Part model, mm, in its own coordinate system. A direction names the side the tool comes from. Round coordinates to 2 decimals unless told otherwise and drop trailing zeros. Write each loop counter-clockwise with the first axis right and the second up, starting at its lowest first coordinate (ties: lowest second). Pieces come first, ordered by that corner, then holes. Notation, with made-up numbers: M -20.5,53.5 L 9.5,53.5 A17 ccw 9.5,62.5 Z; hole C -18,56.25 d11. An arc over 180 degrees is marked long. One line per question, with ' | ' between items. Start each with the question number.
1) Saw through at A-A (y = 97). List the corners of the cut face in (x, z).
2) Saw through at B-B (z = 91.5). List the corners of the cut face in (x, y), plus the area to 3 significant figures.
3) Mould opens along Y. For faces 5 (the face through (110.68, -160.09, 123.18)), 6 (the face through (-1, 158, 124.46)), 7 (the face through (-2, -165.1, 2)) say: pulls with the +Y half, pulls with the -Y half, needs draft (parallel to the pull), parting line crosses it, or undercut.
4) Saw through at C-C (x = 38.5). List the corners of the cut face in (y, z).
5) Drop flat-ended pins along their axis: pin 1 Ø3 at (y, z) = (-39, 125.5) entering from +X; pin 2 Ø1.4 at (x, y) = (112.5, -5) entering from +Z; pin 3 Ø8 at (x, y) = (75, 66) entering from +Z. Give the stop position or say it passes through.
6) Tool access for faces 1 (the face through (-98, -151.1, 125.6)), 2 (the face through (-103.06, -151.12, -45.68)), 3 (the face through (1, 159, 127)), 4 (the face through (110.68, 159.95, 123.18)): list every direction of +Z, -Z, +X, -X, +Y, -Y with a clear straight run to the whole face (end or side of a thin tool).
7) Wall check: probe 1 along Y at (x, z) = (77.5, -93); probe 2 along X at (y, z) = (-65, -15.5); probe 3 along X at (y, z) = (69.5, 112.5). Give the ranges that are in metal, low to high. Write a range as [from, to].
```python
from build123d import *

# Parameters (mm, degrees)
F1_DEPTH      = 165.1
F1_DEPTH_BACK = 165.1
F3_DEPTH      = 12.7
F5_DEPTH      = 5.08
F7_DEPTH      = 5.08
F8_W          = 223.52
F8_H          = 5.08
F9_DEPTH      = 320.04
F11_DEPTH     = 25.4


with BuildPart() as f1:
    # F0 (on Front) → F1 (new body, two sides)
    with BuildSketch(Plane.XZ) as f1_sk:
        with BuildLine():
            Line((-101.6, -127), (101.6, -127))
            ThreePointArc((101.6, -127), (110.580256, -123.280256), (114.3, -114.3))
            Line((114.3, -114.3), (114.3, 114.3))
            ThreePointArc((114.3, 114.3), (110.580256, 123.280256), (101.6, 127))
            Line((101.6, 127), (-101.6, 127))
            ThreePointArc((-101.6, 127), (-110.580256, 123.280256), (-114.3, 114.3))
            Line((-114.3, 114.3), (-114.3, -114.3))
            ThreePointArc((-114.3, -114.3), (-110.580256, -123.280256), (-101.6, -127))
        make_face()
        with BuildLine():
            ThreePointArc((111.76, -111.76), (108.040256, -120.740256), (99.06, -124.46))
            Line((99.06, -124.46), (-99.06, -124.46))
            ThreePointArc((-99.06, -124.46), (-108.040256, -120.740256), (-111.76, -111.76))
            Line((-111.76, -111.76), (-111.76, 111.76))
            ThreePointArc((-111.76, 111.76), (-108.040256, 120.740256), (-99.06, 124.46))
            Line((-99.06, 124.46), (99.06, 124.46))
            ThreePointArc((99.06, 124.46), (108.040256, 120.740256), (111.76, 111.76))
            Line((111.76, 111.76), (111.76, -111.76))
        make_face(mode=Mode.SUBTRACT)
    extrude(amount=F1_DEPTH)
    extrude(f1_sk.sketch, amount=-F1_DEPTH_BACK)

    # F2 (on face) → F3 (cut)
    with BuildSketch(Plane.XY.offset(127)):
        with BuildLine():
            Line((-88.9, -154.94), (312.616626, -154.94))
            Line((312.616626, -154.94), (312.616626, 154.94))
            Line((312.616626, 154.94), (-88.9, 154.94))
            ThreePointArc((-88.9, 154.94), (-97.880256, 151.220256), (-101.6, 142.24))
            Line((-101.6, 142.24), (-101.6, -142.24))
            ThreePointArc((-101.6, -142.24), (-97.880256, -151.220256), (-88.9, -154.94))
        make_face()
    extrude(amount=-F3_DEPTH, mode=Mode.SUBTRACT)

    # F4 (on face) → F5 (join)
    with BuildSketch(Plane.XZ.offset(165.1)):
        with BuildLine():
            Line((-101.6, -127), (101.6, -127))
            ThreePointArc((101.6, -127), (110.580256, -123.280256), (114.3, -114.3))
            Line((114.3, -114.3), (114.3, 114.3))
            ThreePointArc((114.3, 114.3), (110.580256, 123.280256), (101.6, 127))
            Line((101.6, 127), (-101.6, 127))
            ThreePointArc((-101.6, 127), (-110.580256, 123.280256), (-114.3, 114.3))
            Line((-114.3, 114.3), (-114.3, -114.3))
            ThreePointArc((-114.3, -114.3), (-110.580256, -123.280256), (-101.6, -127))
        make_face()
    extrude(amount=-F5_DEPTH)

    # F6 (on face) → F7 (join)
    with BuildSketch(Plane(origin=(0, 165.1, 0), x_dir=(-1, 0, 0), z_dir=(0, 1, 0))):
        with BuildLine():
            Line((-101.6, -127), (101.6, -127))
            ThreePointArc((101.6, -127), (110.580256, -123.280256), (114.3, -114.3))
            Line((114.3, -114.3), (114.3, 114.3))
            ThreePointArc((114.3, 114.3), (110.580256, 123.280256), (101.6, 127))
            Line((101.6, 127), (-101.6, 127))
            ThreePointArc((-101.6, 127), (-110.580256, 123.280256), (-114.3, 114.3))
            Line((-114.3, 114.3), (-114.3, -114.3))
            ThreePointArc((-114.3, -114.3), (-110.580256, -123.280256), (-101.6, -127))
        make_face()
    extrude(amount=-F7_DEPTH)

    # F8 (on face) → F9 (join)
    with BuildSketch(Plane(origin=(0, -160.02, 0), x_dir=(-1, 0, 0), z_dir=(0, 1, 0))):
        with Locations((0, -45.72)):
            Rectangle(F8_W, F8_H)
    extrude(amount=F9_DEPTH)

    # F10 (on face) → F11 (cut)
    with BuildSketch(Plane.XY.offset(-43.18)):
        with BuildLine():
            Line((111.76, -154.94), (111.76, 154.94))
            Line((111.76, 154.94), (-93.98, 154.94))
            ThreePointArc((-93.98, 154.94), (-102.960256, 151.220256), (-106.68, 142.24))
            Line((-106.68, 142.24), (-106.68, -142.24))
            ThreePointArc((-106.68, -142.24), (-102.960256, -151.220256), (-93.98, -154.94))
            Line((-93.98, -154.94), (111.76, -154.94))
        make_face()
    extrude(amount=-F11_DEPTH, mode=Mode.SUBTRACT)


solid = f1.part
```
Answer key:
1) outline: M -114.3,-114.3 A12.7 ccw -101.6,-127 L 101.6,-127 A12.7 ccw 114.3,-114.3 L 114.3,114.3 L 111.5,114.3 A12.7 cw 111.76,111.76 L 111.76,-111.76 A12.7 cw 99.06,-124.46 L -99.06,-124.46 A12.7 cw -111.76,-111.76 L -111.76,-48.26 L -106.68,-48.26 L -106.68,-43.18 L -111.76,-43.18 L -111.76,111.76 A12.7 cw -101.6,124.2 L -101.6,127 A12.7 ccw -114.3,114.3 Z
2) outline: M -114.3,-165.1 L 114.3,-165.1 L 114.3,165.1 L -114.3,165.1 Z; hole M -111.76,-160.02 L 111.76,-160.02 L 111.76,160.02 L -111.76,160.02 Z | area: 3,950 mm2
3) face 5: needs draft | face 6: undercut | face 7: pulls with the -Y half
4) outline: M -165.1,-127 L 165.1,-127 L 165.1,127 L 154.94,127 L 154.94,124.46 L 160.02,124.46 L 160.02,-43.18 L 154.94,-43.18 L 154.94,-48.26 L 160.02,-48.26 L 160.02,-124.46 L -160.02,-124.46 L -160.02,-48.26 L -154.94,-48.26 L -154.94,-43.18 L -160.02,-43.18 L -160.02,124.46 L -154.94,124.46 L -154.94,127 L -165.1,127 Z
5) pin 1: stops at x = -101.6 | pin 2: stops at z = 114.3 | pin 3: stops at z = -124.46
6) face 1: +Z, +X | face 2: none | face 3: +Z, +X, -X, +Y, -Y | face 4: +Z, +X, +Y, -Y
7) probe 1: y = [-165.1, -160.02], [160.02, 165.1] | probe 2: x = [-114.3, -111.76], [111.76, 114.3] | probe 3: x = [-114.3, -111.74], [111.74, 114.3]
